```python
from build123d import *

# Parameters (mm, degrees)
SKETCH1_W               = 141
SKETCH1_H               = 50.1
BOSS_EXTRUDE1_DEPTH     = 0.875
SKETCH3_R               = 1.651
CUT_EXTRUDE1_DEPTH      = 1.875
SKETCH4_R               = 1.75
CUT_EXTRUDE2_DEPTH      = 1.875
CUT_EXTRUDE2_DEPTH_BACK = 1.875
SKETCH2_R               = 5.08
BOSS_EXTRUDE2_DEPTH     = 10.414
BOSS_EXTRUDE3_START     = 0.254
SKETCH5_W               = 7.5
SKETCH5_H               = 3
BOSS_EXTRUDE3_DEPTH     = 6


with BuildPart() as part:
    # Sketch1 → Boss-Extrude1 (new body, symmetric)
    with BuildSketch(Plane(origin=(0, 0, 0), x_dir=(1, 0, 0), z_dir=(0, 1, 0))):
        Rectangle(SKETCH1_W, SKETCH1_H)
    extrude(amount=BOSS_EXTRUDE1_DEPTH, both=True)

    # Sketch3 → Cut-Extrude1 (cut, symmetric)
    with BuildSketch(Plane(origin=(0, 0, 0), x_dir=(1, 0, 0), z_dir=(0, 1, 0))):
        with Locations((67.579, 20.859)):
            Circle(SKETCH3_R)
        with Locations((67.579, -22.199)):
            Circle(SKETCH3_R)
    cut_extrude1 = extrude(amount=CUT_EXTRUDE1_DEPTH, both=True, mode=Mode.SUBTRACT)

    # Sketch4 → Cut-Extrude2 (cut, two sides)
    with BuildSketch(Plane(origin=(0, 0, 0), x_dir=(1, 0, 0), z_dir=(0, 1, 0))) as cut_extrude2_sk:
        with Locations((-57.65, 19.425)):
            Circle(SKETCH4_R)
        with Locations((-15.15, 19.425)):
            Circle(SKETCH4_R)
        with Locations((23.55, 19.425)):
            Circle(SKETCH4_R)
        with Locations((60.2, 19.425)):
            Circle(SKETCH4_R)
        with Locations((-15.15, -3.95)):
            Circle(SKETCH4_R)
        with Locations((23.55, -3.95)):
            Circle(SKETCH4_R)
        with Locations((60.2, -3.95)):
            Circle(SKETCH4_R)
        with Locations((-57.65, -3.95)):
            Circle(SKETCH4_R)
    extrude(amount=CUT_EXTRUDE2_DEPTH, mode=Mode.SUBTRACT)
    extrude(cut_extrude2_sk.sketch, amount=-CUT_EXTRUDE2_DEPTH_BACK, mode=Mode.SUBTRACT)

    # Mirror1: Cut-Extrude1 across plane
    add(cut_extrude1.mirror(Plane(origin=(0, 0, 0), x_dir=(0, 0, 1), z_dir=(1, 0, 0))), mode=Mode.SUBTRACT)

    # Sketch2 → Boss-Extrude2 (add)
    with BuildSketch(Plane(origin=(0, 0.875, 0), x_dir=(1, 0, 0), z_dir=(0, 1, 0))):
        with Locations((-48.5625, 6)):
            Circle(SKETCH2_R)
        with Locations((-31.4175, 6)):
            Circle(SKETCH2_R)
        with Locations((-14.2725, 6)):
            Circle(SKETCH2_R)
        with Locations((0.4595, 6)):
            Circle(SKETCH2_R)
        with Locations((11.3815, 6)):
            Circle(SKETCH2_R)
        with Locations((29.9235, 6)):
            Circle(SKETCH2_R)
        with Locations((46.6875, 6)):
            Circle(SKETCH2_R)
        with Locations((62.5625, 6)):
            Circle(SKETCH2_R)
    extrude(amount=BOSS_EXTRUDE2_DEPTH)

    # Sketch5 → Boss-Extrude3 (add)
    with BuildSketch(Plane.ZY.offset(70.5).offset(BOSS_EXTRUDE3_START)):
        with Locations((13.05, 2.375)):
            Rectangle(SKETCH5_W, SKETCH5_H)
    extrude(amount=-BOSS_EXTRUDE3_DEPTH)


solid = part.part
```
Can you work these out from the model? Positions are in its coordinate system, mm. A direction names the side the tool comes from. Coordinates: 2 decimals unless noted, no trailing zeros. Loops run counter-clockwise (first coordinate to the right, second up) from the corner with the lowest first, then second, coordinate; pieces in that order, holes last.
1) Imagine slicing it at B-B on x = -57.65. List the corners of the cut face in (y, z) for me (3 decimals).
2) Thinking about a two-plate mould opening in Z: for faces 1 (the cylindrical face through (-58.94, 0.01, -20.61)), 2 (the flat face through (-68, 2, 16.8)), 3 (the flat face through (-49, 11.289, -6)), which applies, pulls with the +Z half, pulls with the -Z half, needs draft (parallel to the pull), parting line crosses it, or undercut?
3) Imagine slicing it at C-C on y = 8.5. List the corners of the cut face in (x, z) for me, plus the area to 3 significant figures.
4) For pin 1 (6 mm diameter, centred on x = -51.5, y = 8.5, fed in from -Z); pin 2 (4 mm diameter, centred on x = -67.579, z = -20.859, fed in from +Y) (3 decimals); pin 3 (6.5 mm diameter, centred on x = -68, z = 12.5, fed in from +Y) (3 decimals); pin 4 (3 mm diameter, centred on x = 60.2, z = -19.425, fed in from -Y), each with a flat end and sliding along its axis, tell me the tip position at first contact or that it passes through.
5) Which directions (+Z, -Z, +X, -X, +Y, -Y) give clear straight access to the entire face, cutting with the end or side of a thin tool? Please do faces 4 (the flat face through (-64.754, 2, 13)), 5 (the cylindrical face through (58.91, 0.01, -20.61)), 6 (the flat face through (-70.754, 2, 13)), 7 (the cylindrical face through (-0.202, 6.009, -11.037)), 8 (the flat face through (-68, 2, 9.3)).
6) I need wall thicknesses on probe 1 along Z at (x, y) = (-15.15, 0.15) (3 decimals); probe 2 along X at (y, z) = (-0.5, 3.95); probe 3 along Y at (x, z) = (-21, 21) (3 decimals). Which ranges of each line are inside material? Lowest first, please.
7) Imagine slicing it at D-D on z = 14. List the corners of the cut face in (x, y) for me (3 decimals), plus the area to 3 significant figures.
8) Imagine slicing it at A-A on z = 3.95. List the corners of the cut face in (x, y) for me (3 decimals), plus the area to 3 significant figures.
Completed:
1. outline: (-0.875, -25.05) - (0.875, -25.05) - (0.875, -21.175) - (-0.875, -21.175) - close; (-0.875, -17.675) - (0.875, -17.675) - (0.875, 2.2) - (-0.875, 2.2) - close; (-0.875, 5.7) - (0.875, 5.7) - (0.875, 25.05) - (-0.875, 25.05) - close
2. face 1: undercut
2. face 2: pulls with the +Z half
2. face 3: needs draft
3. outline: circle Ø10.16 at (-48.56, -6); circle Ø10.16 at (-31.42, -6); circle Ø10.16 at (-14.27, -6); circle Ø10.16 at (0.46, -6); circle Ø10.16 at (11.38, -6); circle Ø10.16 at (29.92, -6); circle Ø10.16 at (46.69, -6); circle Ø10.16 at (62.56, -6)
3. area: 649 mm2
4. pin 1: stops at z = -11.08
4. pin 2: stops at y = 0.875
4. pin 3: stops at y = 3.875
4. pin 4: passes through
5. face 4: +Z, -Z, +X, +Y
5. face 5: +Y, -Y
5. face 6: +Z, -Z, -X, +Y, -Y
5. face 7: +Y
5. face 8: -Z, +X, -X, +Y
6. probe 1: z = -25.05 to -21.175, -17.675 to 2.2, 5.7 to 25.05
6. probe 2: x = -70.5 to -59.4, -55.9 to -16.9, -13.4 to 21.8, 25.3 to 58.45, 61.95 to 70.5
6. probe 3: y = -0.875 to 0.875
7. outline: (-70.754, 0.875) - (-70.5, 0.875) - (-70.5, -0.875) - (70.5, -0.875) - (70.5, 0.875) - (-64.754, 0.875) - (-64.754, 3.875) - (-70.754, 3.875) - close
7. area: 265 mm2
8. outline: (-70.5, -0.875) - (-59.4, -0.875) - (-59.4, 0.875) - (-70.5, 0.875) - close; (-55.9, -0.875) - (-16.9, -0.875) - (-16.9, 0.875) - (-55.9, 0.875) - close; (-13.4, -0.875) - (21.8, -0.875) - (21.8, 0.875) - (-13.4, 0.875) - close; (25.3, -0.875) - (58.45, -0.875) - (58.45, 0.875) - (25.3, 0.875) - close; (61.95, -0.875) - (70.5, -0.875) - (70.5, 0.875) - (61.95, 0.875) - close
8. area: 222 mm2
